```python
from build123d import *

# Parameters (mm, degrees)
SKETCH3_R          = 1.5
CUT_EXTRUDE1_DEPTH = 22.975895886


with BuildPart() as part:
    # Sketch1 → Revolve1 (revolve)
    with BuildSketch(Plane(origin=(0, 0, 0), x_dir=(0, 0, -1), z_dir=(1, 0, 0)), mode=Mode.PRIVATE) as revolve1_sk:
        Polygon((6.6, 13), (5.3, 13), (5.3, 14.3), (1.3, 14.3), (1.3, 13), (0, 13), (0, 0), (8.6, 0), (8.6, 3.5), (6.6, 3.5), align=None)
    revolve(revolve1_sk.sketch.rotate(Axis((0, 0, -12.817719844), (0, 0, 1)), 90), axis=Axis((0, 0, -12.817719844), (0, 0, 1)))

    # Sketch3 → Cut-Extrude1 (cut, through all)
    with BuildSketch(Plane.XY):
        Circle(SKETCH3_R)
    extrude(amount=-CUT_EXTRUDE1_DEPTH, mode=Mode.SUBTRACT)


solid = part.part
```
The listing builds one solid part. Answer for the finished solid, in the listing's coordinates (mm). A direction names the side the tool comes from. Coordinates: 2 decimals unless noted, no trailing zeros. Loops run counter-clockwise (first coordinate to the right, second up) from the corner with the lowest first, then second, coordinate; pieces in that order, holes last. Notation, with made-up numbers: M -2.75,41 L 5.25,41 A16 cw 5.25,59 Z; hole C -31,8 d2. An arc over 180 degrees is marked long. Answer as CSV lines item,"result". Start each with the question number.
(1) Given pin 1 (2 mm diameter, centred on x = -2.5, y = -6.5, fed in from -Z); pin 2 (2 mm diameter, centred on x = 7, z = -5.5, fed in from -Y); pin 3 (3 mm diameter, centred on x = 7, z = -6.5, fed in from -Y), each flat-ended and moving along its own axis, determine where each tip first touches the part or whether it passes through.
(2) For faces 4 (the cylindrical face through (10.316, 7.91, -0.641)), 5 (the cylindrical face through (-1.615, 3.105, -7.586)), 6 (the cylindrical face through (1.86, -14.18, -3.27)), determine the directions among +Z, -Z, +X, -X, +Y, -Y from which every point of the face is accessible in a straight line to the end or side of a thin tool.
(3) Find the intervals of material crossed by L1, parallel to Y at x = 0, z = -5.25; L2, parallel to Y at x = 0, z = -6.75; L3, parallel to Z at x = -8.5, y = 2.25, in increasing order. Write a range as [from, to].
(4) The part is cut by section A-A (y = 0). Give the vertices of the cut face in (x, z).
(5) The mould has two halves that part along Y. Classify faces 1 (the cylindrical face through (10.316, 7.91, -5.941)), 2 (the flat face through (3, 13, -5.3)), 3 (the cylindrical face through (-1.5, 0.07, -4.24)): pulls with the +Y half, pulls with the -Y half, needs draft (parallel to the pull), parting line crosses it, or undercut.
(6) The part is cut by section D-D (x = 4.75). Give the vertices of the cut face in (y, z), and give its area (3 significant figures).
(7) The part is cut by section C-C (z = -4.75). Give the vertices of the cut face in (x, y).
Determined:
1,pin 1,"z = -6.6"
1,pin 2,"y = -12.97"
1,pin 3,"y = -12.93"
2,face 4,"+Z"
2,face 5,"-Z"
2,face 6,"+Z, -Z"
3,L1,"[-14.3, -1.5], [1.5, 14.3]"
3,L2,"[-3.5, -1.5], [1.5, 3.5]"
3,L3,"[-6.6, 0]"
4,outline,"M -14.3,-5.3 L -13,-5.3 L -13,-6.6 L -3.5,-6.6 L -3.5,-8.6 L -1.5,-8.6 L -1.5,0 L -13,0 L -13,-1.3 L -14.3,-1.3 Z; M 1.5,-8.6 L 3.5,-8.6 L 3.5,-6.6 L 13,-6.6 L 13,-5.3 L 14.3,-5.3 L 14.3,-1.3 L 13,-1.3 L 13,0 L 1.5,0 Z"
5,face 1,"parting line crosses it"
5,face 2,"needs draft"
5,face 3,"undercut"
6,outline,"M -13.49,-5.3 L -12.1,-5.3 L -12.1,-6.6 L 12.1,-6.6 L 12.1,-5.3 L 13.49,-5.3 L 13.49,-1.3 L 12.1,-1.3 L 12.1,0 L -12.1,0 L -12.1,-1.3 L -13.49,-1.3 Z"
6,area,"171 mm2"
7,outline,"C 0,0 d28.6; hole C 0,0 d3"
